Verification items for the finished model (mm, model axes). Face numbers are marked on the shaded views. A direction names the side the tool comes from. Round coordinates to 2 decimals unless told otherwise and drop trailing zeros. Write each loop counter-clockwise with the first axis right and the second up, starting at its lowest first coordinate (ties: lowest second). Pieces come first, ordered by that corner, then holes. Notation, with made-up numbers: (11, 26) - (47, 26) arc R12 cw to (47, 40) - close; hole circle Ø5 at (37.5, -20). An arc over 180 degrees is marked (long way). Answer as a JSON object with one key per item and string values. Group by question number.
1) Thickness scan on line 1 (X direction, y = -1.75, z = 6.25); line 2 (X direction, y = -11, z = 0.5); line 3 (Y direction, x = 1.5, z = 2.5). Record the ranges inside material, lowest first.
2) Section check B-B (z = 4.5). Enter the section's corners in (x, y), then the cut area to 3 significant figures.
3) Section check A-A (x = 16.25). Enter the section's corners in (y, z).
4) Set-up check for the marked faces 5, 6 and 7: record each of +Z, -Z, +X, -X, +Y, -Y from which the full face is reachable in a straight line by a thin tool's end or side.
5) Section check C-C (y = -2). Enter the section's corners in (x, z), then the cut area to 3 significant figures.
6) Section check D-D (x = 7.25). Enter the section's corners in (y, z).
7) Go/stop test with flat-tipped pins: pin 1 Ø1.1 at (x, y) = (7.5, -0.5) entering from +Z; pin 2 Ø2.5 at (y, z) = (-5, 5.5) entering from +X; pin 3 Ø7.5 at (x, y) = (7.5, -7.5) entering from +Z. Record where each tip stops, or that it passes through.
8) Mould release check, pull along X, two halves, no side actions. Record for the marked faces 1, 2, 3 and 4: +X half, -X half, draft (parallel to the pull), parting line (faces both ways), or undercut.
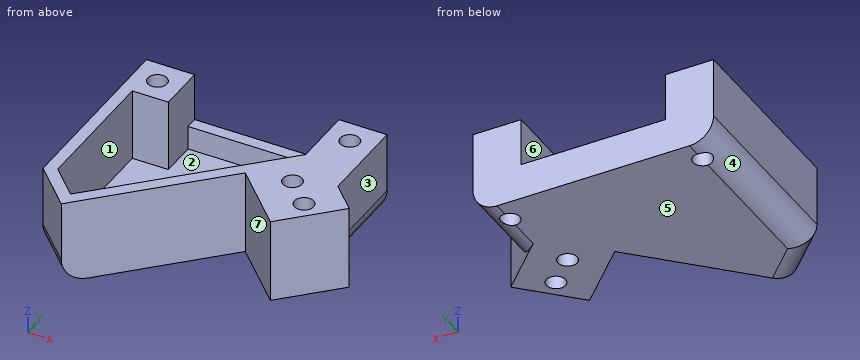
```python
from build123d import *

# Parameters (mm, degrees)
BOSS_EXTRUDE1_DEPTH = 7
BOSS_EXTRUDE2_DEPTH = 1
SKETCH5_R           = 0.799999999
SKETCH5_R_2         = 0.800000001
SCREW_HOLES_DEPTH   = 31.046659105
FILLET1_R           = 2
CUT_EXTRUDE2_START  = 7
SKETCH7_W           = 11.999999998
SKETCH7_H           = 4
CUT_EXTRUDE2_DEPTH  = 4


with BuildPart() as part:
    # Sketch1 → Boss-Extrude1 (new body)
    with BuildSketch(Plane.XY):
        Polygon((0, 0), (19.999999998, 0), (19.999999998, -7.5), (22.085746954, -9.585746956), (17.843106269, -13.828387641), (13.246912191, -9.232193563), (3.347417254, -19.1316885), (0, -15.784271246), align=None)
        Polygon((4, -1), (4, -4), (1, -4), (1, -15.370057685), (3.347417253, -17.717474938), (15.999999998, -5.064892192), (15.999999998, -1), align=None, mode=Mode.SUBTRACT)
    extrude(amount=BOSS_EXTRUDE1_DEPTH)

    # Sketch6 → Boss-Extrude2 (add)
    with BuildSketch(Plane.XY):
        Polygon((0, 0), (19.999999998, 0), (19.999999998, -7.5), (22.085746954, -9.585746956), (17.843106269, -13.828387641), (13.246912191, -9.232193563), (3.347417254, -19.1316885), (0, -15.784271246), align=None)
    extrude(amount=BOSS_EXTRUDE2_DEPTH)

    # Sketch5 → Screw Holes (cut, through all)
    with BuildSketch(Plane.XY):
        with Locations((18.90376644, -10.646407127)):
            Circle(SKETCH5_R)
        with Locations((16.782446096, -8.525086783)):
            Circle(SKETCH5_R)
        with Locations((1.999999999, -2)):
            Circle(SKETCH5_R_2)
        with Locations((17.999999999, -2)):
            Circle(SKETCH5_R_2)
    extrude(amount=SCREW_HOLES_DEPTH, mode=Mode.SUBTRACT)

    # Fillet1
    # the kernel refuses this fillet: 2 mm, written as the material it takes off along each edge
    with BuildSketch(Plane(origin=(19.999999998, 5, 0), x_dir=(-1, 0, 0), z_dir=(0, -1, 0))) as fillet1_piece_1_section:
        with BuildLine():
            CenterArc((FILLET1_R, -FILLET1_R), FILLET1_R, 90, 90)
            Line((0, -FILLET1_R), (0, 0))
            Line((0, 0), (FILLET1_R, 0))
        make_face()
    fillet1_piece_1 = extrude(amount=17.5, mode=Mode.PRIVATE)
    fillet1_piece_1 = split(fillet1_piece_1, bisect_by=Plane(origin=(16.546980954, -4.046980955, 0.4619066), z_dir=(0.7071067811865476, 0.7071067811865476, 0)), keep=Keep.TOP, mode=Mode.PRIVATE)
    add(fillet1_piece_1, mode=Mode.SUBTRACT)
    with BuildSketch(Plane(origin=(6.88295116, -22.667222406, 0), x_dir=(0.7071067811865475, 0.7071067811865477, 0), z_dir=(-0.7071067811865477, 0.7071067811865475, 0))) as fillet1_piece_2:
        with BuildLine():
            CenterArc((FILLET1_R, -FILLET1_R), FILLET1_R, 90, 90)
            Line((0, -FILLET1_R), (0, 0))
            Line((0, 0), (FILLET1_R, 0))
        make_face()
    extrude(amount=14.73396288, mode=Mode.SUBTRACT)
    with BuildSketch(Plane(origin=(0, -20.784271246, 0), x_dir=(1, 0, 0), z_dir=(0, 1, 0))) as fillet1_piece_3:
        with BuildLine():
            CenterArc((FILLET1_R, -FILLET1_R), FILLET1_R, 90, 90)
            Line((0, -FILLET1_R), (0, 0))
            Line((0, 0), (FILLET1_R, 0))
        make_face()
    extrude(amount=25.784271246, mode=Mode.SUBTRACT)

    # Sketch7 → Cut-Extrude2 (cut)
    with BuildSketch(Plane.XY.offset(CUT_EXTRUDE2_START)):
        with Locations((9.999999999, -2)):
            Rectangle(SKETCH7_W, SKETCH7_H)
    extrude(amount=-CUT_EXTRUDE2_DEPTH, mode=Mode.SUBTRACT)


solid = part.part
```
Returned:
{
 "1": {"line 1": "0 to 1.24, 2.76 to 4, 16 to 17.24, 18.76 to 20", "line 2": "0.68 to 11.48, 15.01 to 18.19, 19.62 to 20.67", "line 3": "-17.28 to -15.87, -4 to -2.62, -1.38 to 0"},
 "2": {"outline": "(0, -15.78) - (3.35, -19.13) - (13.25, -9.23) - (17.84, -13.83) - (22.09, -9.59) - (20, -7.5) - (20, 0) - (16, 0) - (16, -5.06) - (3.35, -17.72) - (1, -15.37) - (1, -4) - (4, -4) - (4, 0) - (0, 0) - close; hole circle Ø1.6 at (2, -2); hole circle Ø1.6 at (16.78, -8.53); hole circle Ø1.6 at (18, -2); hole circle Ø1.6 at (18.9, -10.65)", "area": "105 mm2"},
 "3": {"outline": "(-12.24, 0) - (-9.12, 0) - (-9.12, 7) - (-12.24, 7) - close; (-7.93, 0) - (0, 0) - (0, 7) - (-7.93, 7) - close"},
 "4": {"face 5": "-Z, +X, -X, +Y, -Y", "face 6": "+Z", "face 7": "+Z, -Z, -Y"},
 "5": {"outline": "(0, 2) arc R2 ccw to (1.2, 0.17) - (1.2, 7) - (0, 7) - close; (2.8, 0) - (17.2, 0) - (17.2, 7) - (16, 7) - (16, 1) - (4, 1) - (4, 7) - (2.8, 7) - close; (18.8, 0.17) arc R2 ccw to (20, 2) - (20, 7) - (18.8, 7) - close", "area": "44.0 mm2"},
 "6": {"outline": "(-15.23, 0) - (0, 0) - (0, 3) - (-1, 3) - (-1, 1) - (-13.81, 1) - (-13.81, 7) - (-15.23, 7) - close"},
 "7": {"pin 1": "z = 3", "pin 2": "x = 20", "pin 3": "z = 1"},
 "8": {"face 1": "undercut", "face 2": "undercut", "face 3": "+X half", "face 4": "-X half"}
}
